from build123d import *

# Parameters (mm, degrees)
SKETCH1_W           = 60
SKETCH1_H           = 166
BOSS_EXTRUDE1_DEPTH = 5
SKETCH2_W           = 50
SKETCH2_H           = 50
BOSS_EXTRUDE3_DEPTH = 2
LPATTERN1_COUNT     = 3
LPATTERN1_PITCH     = 52
SKETCH3_W           = 52
SKETCH3_H           = 51.9
BOSS_EXTRUDE8_DEPTH = 25
LPATTERN5_COUNT     = 3
LPATTERN5_PITCH     = 52


with BuildPart() as part:
    # Sketch1 → Boss-Extrude1 (new body)
    with BuildSketch(Plane(origin=(0, 0, 0), x_dir=(1, 0, 0), z_dir=(0, 1, 0))):
        Rectangle(SKETCH1_W, SKETCH1_H)
    extrude(amount=BOSS_EXTRUDE1_DEPTH)

    # Sketch2 → Boss-Extrude3 (add)
    with BuildSketch(Plane(origin=(0, 5, 0), x_dir=(1, 0, 0), z_dir=(0, 1, 0))):
        with Locations((0, -53)):
            Rectangle(SKETCH2_W, SKETCH2_H)
    boss_extrude3 = extrude(amount=BOSS_EXTRUDE3_DEPTH)

    # LPattern1: Boss-Extrude3 ×3
    with Locations(*[(0, 0, -i * LPATTERN1_PITCH) for i in range(1, LPATTERN1_COUNT)]):
        add(boss_extrude3)

    # Sketch3 → Boss-Extrude8 (add)
    with BuildSketch(Plane(origin=(0, 7, 0), x_dir=(1, 0, 0), z_dir=(0, 1, 0))):
        with Locations((0, -53.05)):
            Rectangle(SKETCH3_W, SKETCH3_H)
    boss_extrude8 = extrude(amount=BOSS_EXTRUDE8_DEPTH)

    # LPattern5: Boss-Extrude8 ×3
    with Locations(*[(0, 0, -i * LPATTERN5_PITCH) for i in range(1, LPATTERN5_COUNT)]):
        add(boss_extrude8)


solid = part.part
Read the model definition and answer for the solid it produces. Units are mm, in the model's axes. A direction names the side the tool comes from. Coordinates: 2 decimals unless noted, no trailing zeros. Loops run counter-clockwise (first coordinate to the right, second up) from the corner with the lowest first, then second, coordinate; pieces in that order, holes last. Notation, with made-up numbers: (56.5, -23.75) -> (112.5, -23.75) arc R19 ccw to (112.5, -7.75) -> close; hole circle Ø6 at (-8.5, 52.25). An arc over 180 degrees is marked (long way). Answer in a Markdown table with one row per item.
Item 1: A cutting plane is placed at C-C on z = -13. Determine the outline of the cut face in (x, y).
Returned:
| item | result |
|---|---|
| outline | (-30, 0) -> (30, 0) -> (30, 5) -> (25, 5) -> (25, 7) -> (26, 7) -> (26, 32) -> (-26, 32) -> (-26, 7) -> (-25, 7) -> (-25, 5) -> (-30, 5) -> close |
Item 2: Each of these flat-tipped pins is pushed along its axis until it touches: P1, Ø1.5, axis at x = 4.5, y = 25.5, coming from the -Z side; P2, Ø0.6, axis at x = -5, y = 6.5, coming from the +Z side; P3, Ø1, axis at y = 6, z = -44, coming from the -X side. Where does it stop, or does it pass through?
Returned:
| item | result |
|---|---|
| P1 | stops at z = -76.9 |
| P2 | stops at z = 78 |
| P3 | stops at x = -25 |
Item 3: Straight lines are drawn through the part: line 1 along Y through (x, z) = (-25.5, 1); line 2 along X through (y, z) = (23.5, -53). For each, find the intervals that lie inside material, in ascending order. Write a range as [from, to].
Returned:
| item | result |
|---|---|
| line 1 | y = [0, 5], [7, 32] |
| line 2 | x = [-26, 26] |
Item 4: A cutting plane is placed at B-B on x = 22. Determine the outline of the cut face in (y, z).
Returned:
| item | result |
|---|---|
| outline | (0, -83) -> (5, -83) -> (5, -76) -> (7, -76) -> (7, -76.9) -> (32, -76.9) -> (32, -25) -> (7, -25) -> (7, -26) -> (5, -26) -> (5, -24) -> (7, -24) -> (7, -24.9) -> (32, -24.9) -> (32, 27) -> (7, 27) -> (7, 26) -> (5, 26) -> (5, 28) -> (7, 28) -> (7, 27.1) -> (32, 27.1) -> (32, 79) -> (7, 79) -> (7, 78) -> (5, 78) -> (5, 83) -> (0, 83) -> close |
Item 5: For faces 4 (the flat face through (0, 19, 79)), 5 (the flat face through (-26, 19, 1)), 6 (the flat face through (0, 32, 1)), 7 (the flat face through (0, 2, -83)), 8 (the flat face through (26, 19, 1)), determine the directions among +Z, -Z, +X, -X, +Y, -Y from which every point of the face is accessible in a straight line to the end or side of a thin tool.
Returned:
| item | result |
|---|---|
| face 4 | +Z, +X, -X, +Y |
| face 5 | +Z, -Z, -X, +Y |
| face 6 | +Z, -Z, +X, -X, +Y |
| face 7 | -Z, +X, -X, +Y, -Y |
| face 8 | +Z, -Z, +X, +Y |
Item 6: For a pull along Z with two mould halves and no side action, classify faces 1 (the flat face through (26, 19, -51)), 2 (the flat face through (0, 2, 83)), 3 (the flat face through (-25.2, 7, -10.6)) as released by +Z, released by -Z, zero draft, split by the parting line, or undercut.
Returned:
| item | result |
|---|---|
| face 1 | zero draft |
| face 2 | released by +Z |
| face 3 | undercut |
Item 7: A cutting plane is placed at A-A on y = 15. Determine the outline of the cut face in (x, z).
Returned:
| item | result |
|---|---|
| outline | (-26, -76.9) -> (26, -76.9) -> (26, -25) -> (-26, -25) -> close; (-26, -24.9) -> (26, -24.9) -> (26, 27) -> (-26, 27) -> close; (-26, 27.1) -> (26, 27.1) -> (26, 79) -> (-26, 79) -> close |
